Geometry check sheet. Reference: the model listing, model coordinates, mm. Face numbers are marked on the shaded views. Give positions to 0.01 mm unless a question says otherwise; leave off trailing zeros. Write each loop counter-clockwise with the first axis right and the second up, starting at its lowest first coordinate (ties: lowest second). Pieces come first, ordered by that corner, then holes. Notation, with made-up numbers: (43, 57.5) - (67, 57.5) arc R17 ccw to (67, 75.5) - close; hole circle Ø7 at (-7.75, 41). An arc over 180 degrees is marked (long way). Write item = value, one per line. Start each with the question number.
(1) Section check B-B, the plane y = -11. Enter the section's corners in (x, z).
(2) Thickness scan on L1, parallel to Y at x = 0, z = 0.65; L2, parallel to X at y = 0, z = 35; L3, parallel to Z at x = -7, y = 15. Record the ranges inside material, lowest first.
(3) Draft check along Y on the marked faces 1, 2 and 3. Enter one of: pulls with the +Y half, pulls with the -Y half, needs draft (parallel to the pull), parting line crosses it, or undercut.
(4) Section check A-A, the plane x = 0. Enter the section's corners in (y, z).
(5) Section check C-C, the plane y = 0. Enter the section's corners in (x, z), plus the area to 3 significant figures.
(6) Depth check by flat-ended pin: pin 1 Ø8 at (y, z) = (11.5, 74) entering from +X; pin 2 Ø12 at (x, z) = (-0.5, 71) entering from +Y; pin 3 Ø10 at (y, z) = (-7, 26.5) entering from +X. Enter the tip coordinate at first touch or a pass-through.
(7) Section check D-D, the plane x = -16. Enter the section's corners in (y, z), plus the area to 3 significant figures.
```python
from build123d import *

# Parameters (mm, degrees)
F2_T     = -1.27
F3_DEPTH = 1.27
F5_R     = 19.685
F6_DEPTH = 25.4
F7_W     = 1.905
F7_H     = 19.812
F8_DEPTH = 76.2
F9_W     = 2.54
F9_H     = 2.54


with BuildPart() as f1:
    # F0 (on Front) → F1 (revolve)
    with BuildSketch(Plane.XZ):
        Polygon((0, 2.54), (0, 0), (21.082, 0), (21.082, 88.9), (0, 88.9), align=None)
        Polygon((0, 91.44), (0, 88.9), (21.082, 88.9), (25.4, 88.9), (25.4, 91.44), align=None)
    revolve(axis=Axis((0, 0, 44.45), (0, 0, 1)))

    # F2
    f2_openings = [f1.faces().sort_by_distance(p)[0] for p in [
        (0, 0, 91.44),
    ]]
    offset(amount=F2_T, openings=f2_openings, kind=Kind.INTERSECTION)

    # F3 (add): a face of the model
    f3_faces = [f1.faces().sort_by_distance(p)[0] for p in [
        (-23.4475005348, 0, 90.17),
    ]]
    extrude(f3_faces, amount=F3_DEPTH)

    # F5 (on offset) → F6 (cut)
    with BuildSketch(Plane.XY.offset(88.9)):
        Circle(F5_R)
    extrude(amount=F6_DEPTH, mode=Mode.SUBTRACT)

    # F7 (on Top) → F8 (cut)
    with BuildSketch(Plane.XY):
        Polygon((0.9525, -27.178), (0.9525, -7.366), (0, -7.366), (-0.9525, -7.366), (-0.9525, -27.178), align=None)
        Polygon((5.2068558942, -5.3647039539), (3.6656785199, -6.4844348595), (15.3108799383, -22.5126795521), (16.8520573126, -21.3929486464), align=None)
        Polygon((7.4723698113, -1.2449737892), (6.883692437, -3.0567364527), (25.7260241378, -9.1789811453), (26.3147015121, -7.3672184818), align=None)
        Polygon((6.883692437, 3.4195935956), (7.4723698113, 1.6078309321), (26.3147015121, 7.7300756246), (25.7260241378, 9.5418382882), align=None)
        Polygon((3.6656785199, 6.8472920024), (5.2068558942, 5.7275610967), (16.8520573126, 21.7558057893), (15.3108799383, 22.8755366949), align=None)
        with Locations((0, 17.6348571429)):
            Rectangle(F7_W, F7_H)
        Polygon((-5.2068558942, 5.7275610967), (-3.6656785199, 6.8472920024), (-15.3108799383, 22.8755366949), (-16.8520573126, 21.7558057893), align=None)
        Polygon((-7.4723698113, 1.6078309321), (-6.883692437, 3.4195935956), (-25.7260241378, 9.5418382882), (-26.3147015121, 7.7300756246), align=None)
        Polygon((-6.883692437, -3.0567364527), (-7.4723698113, -1.2449737892), (-26.3147015121, -7.3672184818), (-25.7260241378, -9.1789811453), align=None)
        Polygon((-3.6656785199, -6.4844348595), (-5.2068558942, -5.3647039539), (-16.8520573126, -21.3929486464), (-15.3108799383, -22.5126795521), align=None)
    extrude(amount=F8_DEPTH, mode=Mode.SUBTRACT)

    # F9 (on Front) → F10 (revolve)
    with BuildSketch(Plane.XZ):
        with Locations((19.812, 1.27)):
            Rectangle(F9_W, F9_H)
    revolve(axis=Axis((0, 0, 1.27), (0, 0, 1)))


solid = f1.part
```
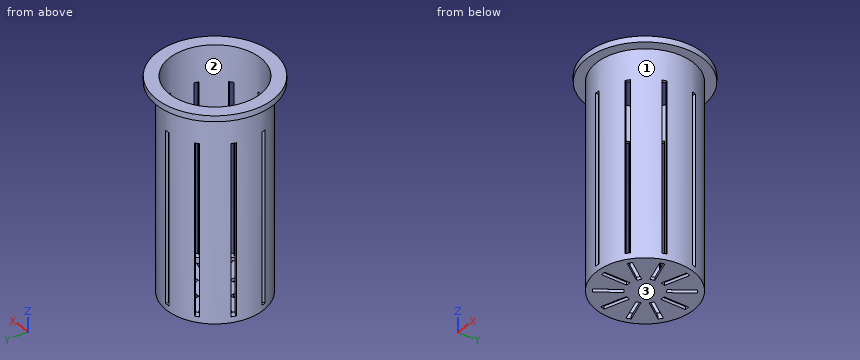
Model answer:
q1.outline = (-22.89, 88.9) - (-17.98, 88.9) - (-17.98, 0) - (-9.3, 0) - (-9.3, 1.27) - (-14.93, 1.27) - (-14.93, 2.54) - (-16.48, 2.54) - (-16.48, 91.44) - (-22.89, 91.44) - close; (-6.95, 0) - (-0.95, 0) - (-0.95, 1.27) - (-6.95, 1.27) - close; (0.95, 0) - (6.95, 0) - (6.95, 1.27) - (0.95, 1.27) - close; (9.3, 0) - (17.98, 0) - (17.98, 88.9) - (22.89, 88.9) - (22.89, 91.44) - (16.48, 91.44) - (16.48, 2.54) - (14.93, 2.54) - (14.93, 1.27) - (9.3, 1.27) - close
q2.L1 = -21.08 to -18.54, -7.37 to 7.73, 18.54 to 21.08
q2.L2 = -21.08 to -19.81, 19.81 to 21.08
q2.L3 = 0 to 1.27
q3.face_1 = parting line crosses it
q3.face_2 = undercut
q3.face_3 = needs draft
q4.outline = (-25.4, 88.9) - (-21.08, 88.9) - (-21.08, 76.2) - (-19.81, 76.2) - (-19.81, 91.44) - (-25.4, 91.44) - close; (-21.08, 0) - (-18.54, 0) - (-18.54, 2.54) - (-21.08, 2.54) - close; (-7.37, 0) - (7.73, 0) - (7.73, 1.27) - (-7.37, 1.27) - close; (18.54, 0) - (21.08, 0) - (21.08, 2.54) - (18.54, 2.54) - close; (19.81, 76.2) - (21.08, 76.2) - (21.08, 88.9) - (25.4, 88.9) - (25.4, 91.44) - (19.81, 91.44) - close
q5.outline = (-25.4, 88.9) - (-21.08, 88.9) - (-21.08, 0) - (21.08, 0) - (21.08, 88.9) - (25.4, 88.9) - (25.4, 91.44) - (19.81, 91.44) - (19.81, 2.54) - (18.54, 2.54) - (18.54, 1.27) - (-18.54, 1.27) - (-18.54, 2.54) - (-19.81, 2.54) - (-19.81, 91.44) - (-25.4, 91.44) - close
q5.area = 308 mm²
q6.pin_1 = 19.67
q6.pin_2 = 21.08
q6.pin_3 = 20.99
q7.outline = (-19.73, 88.9) - (-13.73, 88.9) - (-13.73, 0) - (-6.02, 0) - (-6.02, 1.27) - (-9.37, 1.27) - (-9.37, 2.54) - (-11.68, 2.54) - (-11.68, 91.44) - (-19.73, 91.44) - close; (-4.02, 0) - (4.38, 0) - (4.38, 1.27) - (-4.02, 1.27) - close; (6.38, 0) - (13.73, 0) - (13.73, 88.9) - (19.73, 88.9) - (19.73, 91.44) - (11.68, 91.44) - (11.68, 2.54) - (9.37, 2.54) - (9.37, 1.27) - (6.38, 1.27) - close
q7.area = 435 mm²
